from build123d import *

# Parameters (mm, degrees)
F1_DEPTH    = 25.4
F3_R        = 10.16
F2_R        = 6.35
F4_DEPTH    = 26.7233065934
F6_DEPTH    = 26.7232814104
F7_T1_DEPTH = 66.7645981405
F7_T3_DEPTH = 66.7279267596
F9_DEPTH    = 50.8


# Not quite as in the source:
# - a fillet or chamfer that OpenCascade refuses, or shapes differently, is made with other operations: its cross-section is extruded or revolved along the edge and cut away or added


with BuildPart() as f1:
    # F0 (on Front) → F1 (new body)
    with BuildSketch(Plane.XZ):
        Polygon((27.0092859864, -6.985), (19.05, -6.985), (0, -6.985), (0, -13.335), (38.1, -13.335), (38.1, 13.3873065934), (0, 13.335), (0, 6.985), (19.05, 6.985), (27.0092859864, 6.985), align=None)
    extrude(amount=F1_DEPTH)

    # F3
    f3_edges = [f1.edges().sort_by_distance(p)[0] for p in [
        (0, 0, -10.16),
        (0, 0, 10.16),
        (0, -25.4, 10.16),
        (0, -25.4, -10.16),
    ]]
    fillet(f3_edges, radius=F3_R)

    # F2 (on face) → F4 (cut, through all)
    with BuildSketch(Plane(origin=(0, 0, -13.335), x_dir=(1, 0, 0), z_dir=(0, 0, -1))):
        with Locations((8.1856111065, 12.7)):
            Circle(F2_R)
    extrude(amount=-F4_DEPTH, mode=Mode.SUBTRACT)

    # F5 (on face) → F6 (cut, through all)
    with BuildSketch(Plane(origin=(-0.0183072732, 0, 13.3349748664), x_dir=(0.9999990576, 0, 0.0013728752), z_dir=(-0.0013728752, 0, 0.9999990576))):
        with BuildLine():
            Line((20.423270762, 6.0135265812), (-7.3266747168, -5.8177547927))
            Line((-7.3266747168, -5.8177547927), (0.9929662687, -5.8177547927))
            add(Edge.make_bspline(
                [(10.1783168652, 0), (3.7432331436, 0), (0.9929662687, -5.8177547927)],
                knots=[4.7123889804, 4.7123889804, 4.7123889804, 5.8269772874, 5.8269772874, 5.8269772874], degree=2, weights=[1, 0.792172065, 0.879280631]))
            Line((10.1783168652, 0), (22.1537450551, 0))
            Line((22.1537450551, 0), (20.423270762, 6.0135265812))
        make_face()
        with BuildLine():
            add(Edge.make_bspline(
                [(10.1783168652, 0), (3.7432331436, 0), (0.9929662687, -5.8177547927)],
                knots=[4.7123889804, 4.7123889804, 4.7123889804, 5.8269772874, 5.8269772874, 5.8269772874], degree=2, weights=[1, 0.792172065, 0.879280631]))
            Line((0.9929662687, -5.8177547927), (22.1537450551, -5.8177547927))
            Line((22.1537450551, -5.8177547927), (22.1537450551, 0))
            Line((22.1537450551, 0), (10.1783168652, 0))
        make_face()
        with BuildLine():
            Line((22.1537450551, -25.4), (22.1537450551, -19.5822452073))
            Line((22.1537450551, -19.5822452073), (0.9929662687, -19.5822452073))
            add(Edge.make_bspline(
                [(0.9929662687, -19.5822452073), (3.7432331436, -25.4), (10.1783168652, -25.4)],
                knots=[0.4562080198, 0.4562080198, 0.4562080198, 1.5707963268, 1.5707963268, 1.5707963268], degree=2, weights=[0.879280631, 0.792172065, 1]))
            Line((10.1783168652, -25.4), (22.1537450551, -25.4))
        make_face()
        with BuildLine():
            Line((0.9929662687, -19.5822452073), (-6.3022147662, -19.5822452073))
            Line((-6.3022147662, -19.5822452073), (17.9763548076, -30.6573584676))
            Line((17.9763548076, -30.6573584676), (22.1537450551, -25.4))
            Line((22.1537450551, -25.4), (10.1783168652, -25.4))
            add(Edge.make_bspline(
                [(0.9929662687, -19.5822452073), (3.7432331436, -25.4), (10.1783168652, -25.4)],
                knots=[0.4562080198, 0.4562080198, 0.4562080198, 1.5707963268, 1.5707963268, 1.5707963268], degree=2, weights=[0.879280631, 0.792172065, 1]))
        make_face()
    extrude(amount=-F6_DEPTH, mode=Mode.SUBTRACT)

    # F7: fillet of radius 10.16 on 4 edges, made by hand

    # F7_s2 → F7_t1 (cut)
    with BuildSketch(Plane(origin=(63.5182833364, 0, 0.0872027564), x_dir=(0, 1, 0), z_dir=(-0.9999990576, 0, -0.0013728752))):
        with BuildLine():
            ThreePointArc((-25.4, -3.1749874332), (-22.4242048969, -10.35919233), (-15.24, -13.3349874332))
            Line((-15.24, -13.3349874332), (-25.4, -13.3349874332))
            Line((-25.4, -13.3349874332), (-25.4, -3.1749874332))
        make_face()
        with BuildLine():
            ThreePointArc((0, -3.1749874332), (-2.9757951031, -10.35919233), (-10.16, -13.3349874332))
            Line((-10.16, -13.3349874332), (0, -13.3349874332))
            Line((0, -13.3349874332), (0, -3.1749874332))
        make_face()
    extrude(amount=F7_T1_DEPTH, mode=Mode.SUBTRACT)

    # F7_s4 → F7_t3 (cut)
    with BuildSketch(Plane.YZ.offset(-3.2279267596)):
        with BuildLine():
            ThreePointArc((0, -3.175), (-2.9757951031, -10.3592048969), (-10.16, -13.335))
            Line((-10.16, -13.335), (0, -13.335))
            Line((0, -13.335), (0, -3.175))
        make_face()
        with BuildLine():
            ThreePointArc((-25.4, -3.175), (-22.4242048969, -10.3592048969), (-15.24, -13.335))
            Line((-15.24, -13.335), (-25.4, -13.335))
            Line((-25.4, -13.335), (-25.4, -3.175))
        make_face()
    extrude(amount=F7_T3_DEPTH, mode=Mode.SUBTRACT)

    # F8 (on Top) → F9 (cut, symmetric)
    with BuildSketch(Plane.XY):
        Polygon((-2.6969234459, -10.516657494), (6.3479291275, -5.0737368874), (-5.7385554537, -5.0737368874), (-5.7385554537, -20.2818978578), (6.3479291275, -20.2818978578), (-2.6969234459, -14.9190193042), align=None)
    extrude(amount=F9_DEPTH, both=True, mode=Mode.SUBTRACT)


solid = f1.part
Here's how the part is built. I have some questions about the finished solid (model axes, mm). A direction names the side the tool comes from. Give positions to 0.01 mm unless a question says otherwise; leave off trailing zeros. Order: outer loops, then holes, each group sorted by start corner. A loop starts at its lowest first (then second) coordinate and runs counter-clockwise, first axis right, second up. Notation, with made-up numbers: M 23.5,-16.75 L 70.5,-16.75 A11 ccw 70.5,-9.75 Z; hole C -32,-23 d9. An arc over 180 degrees is marked long. Answer as a JSON object with one key per item and string values. Group by question number.
1) Suppose I cut it at A-A, the plane y = -7.5. Write out the boundary of the cut face in (x, z) (3 decimals), plus the area to 3 significant figures.
2) I'm going to push flat-ended pins straight in: pin 1 Ø1 at (x, z) = (34, 7.5) entering from -Y; pin 2 Ø1.5 at (x, y) = (18, -13) entering from +Z; pin 3 Ø5 at (x, y) = (11, -9) entering from -Z; pin 4 Ø10 at (x, y) = (8.19, -12.7) entering from -Z. Where does each tip first touch, or does it pass through?
3) Suppose I cut it at B-B, the plane z = -9.25. Write out the boundary of the cut face in (x, y), plus the area to 3 significant figures.
4) Please list where these lines run through material, in increasing order: L1, parallel to X at y = -12.7, z = -12; L2, parallel to Z at x = 16, y = -13.75 (3 decimals); L3, parallel to X at y = -5.5, z = -2. Write a range as [from, to].
5) On a 3-axis mill with a long thin cutter (end or side, diameter ignored), from which of +Z, -Z, +X, -X, +Y, -Y can I reach the whole of each face in a straight line? I mean faces 1 (the flat face through (14, -5.818, 10)), 2 (the flat face through (32, -25.4, 0)), 3 (the flat face through (27.009, -13, 0)). Say none if no direction works.
6) Suppose I cut it at C-C, the plane x = 10. Count the separate pieces of the cut face and the enclosed holes in it, plus the area to 3 significant figures.
7) Suppose I cut it at D-D, the plane y = -12.7. Write out the boundary of the cut face in (x, z) (3 decimals), plus the area to 3 significant figures.
8) We'd pull the mould along Y, two halves only. Please class faces 4 (the flat face through (0, -13, 10)), 5 (the flat face through (14, -5.818, -10)), 6 (the flat face through (14, -19.582, 10)), 7 (the cylindrical face through (1.84, -12.98, -10.2)): pulls with the +Y half, pulls with the -Y half, needs draft (parallel to the pull), parting line crosses it, or undercut.
Results found:
{
 "1": {"outline": "M 2.316,-12.981 L 4.541,-12.981 L 4.541,-6.985 L 2.316,-6.985 Z; M 2.316,6.985 L 4.541,6.985 L 4.541,12.987 L 2.316,12.984 Z; M 11.83,-12.981 L 38.1,-12.981 L 38.1,13.033 L 11.83,12.997 L 11.83,6.985 L 27.009,6.985 L 27.009,-6.985 L 11.83,-6.985 Z", "area": "498 mm²"},
 "2": {"pin 1": "y = -24.67", "pin 2": "z = 13.36", "pin 3": "z = -13.29", "pin 4": "through"},
 "3": {"outline": "M 0,-15.24 A10.16 ccw 0.09,-16.57 L 5.17,-19.58 L 22.17,-19.58 L 22.17,-23.38 L 38.1,-23.38 L 38.1,-2.02 L 22.17,-2.02 L 22.17,-5.82 L 5.11,-5.82 L 0.09,-8.84 A10.16 ccw 0,-10.16 Z; hole C 8.19,-12.7 d12.7", "area": "503 mm²"},
 "4": {"L1": "[0, 1.84], [14.54, 38.1]", "L2": "[-13.335, -6.985], [6.985, 13.357]", "L3": "[27.01, 38.1]"},
 "5": {"face 1": "+Z, -Z, -X, +Y", "face 2": "+Z, -Z, +X, -X, -Y", "face 3": "-X, +Y, -Y"},
 "6": {"separate pieces": "4", "enclosed holes": "0", "area": "17.7 mm²"},
 "7": {"outline": "M 0,-13.335 L 1.836,-13.335 L 1.836,-6.985 L 0,-6.985 Z; M 0,6.985 L 1.836,6.985 L 1.836,13.338 L 0,13.335 Z; M 14.536,-13.335 L 38.1,-13.335 L 38.1,13.387 L 14.536,13.355 L 14.536,6.985 L 27.009,6.985 L 27.009,-6.985 L 14.536,-6.985 Z", "area": "478 mm²"},
 "8": {"face 4": "needs draft", "face 5": "pulls with the +Y half", "face 6": "pulls with the -Y half", "face 7": "undercut"}
}
